```python
from build123d import *

# Parameters (mm, degrees)
F0_W     = 165.1
F0_H     = 139.7
F1_DEPTH = 12.7
F2_D     = 6.8
F3_D     = 5
F4_D     = 4


with BuildPart() as f1:
    # F0 (on Top) → F1 (new body)
    with BuildSketch(Plane.XY):
        Rectangle(F0_W, F0_H)
    extrude(amount=F1_DEPTH)

    # F2 (through all)
    with Locations(Plane(origin=(0, 0, 0), x_dir=(1, 0, 0), z_dir=(0, 0, -1))):
        with Locations((-58, -18.8), (0, -61), (58, -18.8), (35.8, 49.3), (-35.8, 49.3)):
            Hole(F2_D / 2)

    # F3 (through all)
    with Locations(Plane(origin=(0, 0, 0), x_dir=(1, 0, 0), z_dir=(0, 0, -1))):
        with Locations((-71.418902627, 27.4151481402), (-75.9297806006, 9.3230047705), (-75.9297806006, -9.3230047705), (-71.418902627, -27.4151481402), (71.418902627, 27.4151481402), (75.9297806006, 9.3230047705), (75.9297806006, -9.3230047705), (71.418902627, -27.4151481402)):
            Hole(F3_D / 2)

    # F4 (through all)
    with Locations(Plane(origin=(0, 0, 0), x_dir=(1, 0, 0), z_dir=(0, 0, -1))):
        with Locations((0, 0)):
            Hole(F4_D / 2)


solid = f1.part
```
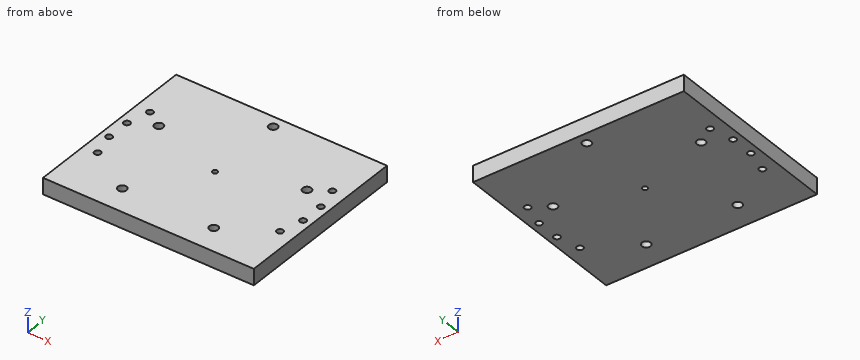
Model file for the job. Use its own axes, mm. Coordinates: 2 decimals unless noted, no trailing zeros. Loops run counter-clockwise (first coordinate to the right, second up) from the corner with the lowest first, then second, coordinate; pieces in that order, holes last. Notation, with made-up numbers: (-5.75, 64.25) - (49.25, 64.25) arc R25 cw to (49.25, 86.25) - close; hole circle Ø2 at (60, 56). An arc over 180 degrees is marked (long way). Write item = value, one per line. Start each with the question number.
Item 1: Saw through at C-C, the plane x = 0. List the corners of the cut face in (y, z), then the cut area to 3 significant figures.
Item 2: Saw through at D-D, the plane y = 18.8. List the corners of the cut face in (x, z), then the cut area to 3 significant figures.
Item 3: Wall check: probe 1 along X at (y, z) = (18.8, 7); probe 2 along X at (y, z) = (-49.3, 6.25); probe 3 along X at (y, z) = (60.5, 4). Give the ranges that are in metal, low to high. Write a range as [from, to].
Item 4: Saw through at B-B, the plane x = -58. List the corners of the cut face in (y, z), then the cut area to 3 significant figures.
Item 5: Saw through at A-A, the plane y = 61. List the corners of the cut face in (x, z).
Answers:
q1.outline = (-69.85, 0) - (-2, 0) - (-2, 12.7) - (-69.85, 12.7) - close; (2, 0) - (57.6, 0) - (57.6, 12.7) - (2, 12.7) - close; (64.4, 0) - (69.85, 0) - (69.85, 12.7) - (64.4, 12.7) - close
q1.area = 1,640 mm2
q2.outline = (-82.55, 0) - (-61.4, 0) - (-61.4, 12.7) - (-82.55, 12.7) - close; (-54.6, 0) - (54.6, 0) - (54.6, 12.7) - (-54.6, 12.7) - close; (61.4, 0) - (82.55, 0) - (82.55, 12.7) - (61.4, 12.7) - close
q2.area = 1,920 mm2
q3.probe_1 = [-82.55, -61.4], [-54.6, 54.6], [61.4, 82.55]
q3.probe_2 = [-82.55, -39.2], [-32.4, 32.4], [39.2, 82.55]
q3.probe_3 = [-82.55, -3.36], [3.36, 82.55]
q4.outline = (-69.85, 0) - (15.4, 0) - (15.4, 12.7) - (-69.85, 12.7) - close; (22.2, 0) - (69.85, 0) - (69.85, 12.7) - (22.2, 12.7) - close
q4.area = 1,690 mm2
q5.outline = (-82.55, 0) - (-3.4, 0) - (-3.4, 12.7) - (-82.55, 12.7) - close; (3.4, 0) - (82.55, 0) - (82.55, 12.7) - (3.4, 12.7) - close
